Geometry check sheet. Reference: the model listing, model coordinates, mm. A direction names the side the tool comes from. Coordinates: 2 decimals unless noted, no trailing zeros. Loops run counter-clockwise (first coordinate to the right, second up) from the corner with the lowest first, then second, coordinate; pieces in that order, holes last. Notation, with made-up numbers: (-31.5, 16.5) - (3.5, 16.5) arc R9 cw to (3.5, 33.5) - close; hole circle Ø8 at (38, -34). An arc over 180 degrees is marked (long way). Write each question's results on one line, items separated by ' | '. Start each with the question number.
(1) Go/stop test with flat-tipped pins: pin 1 Ø6 at (x, y) = (17.5, 1) entering from -Z; pin 2 Ø5 at (x, y) = (-27.6, 8.005) entering from -Z; pin 3 Ø5 at (x, y) = (-27.6, -8.005) entering from +Z; pin 4 Ø3.5 at (x, y) = (27.6, 8.005) entering from -Z. Record where each tip stops, or that it passes through.
(2) Sectioned sample at B-B (z = 2.75). Enter the section's corners in (x, y).
(3) Sectioned sample at C-C (x = 31.5). Enter the section's corners in (y, z) (3 decimals).
(4) Material ranges on probe 1 along Y at (x, z) = (27.6, 1.35) (3 decimals); probe 2 along X at (y, z) = (-3, 15.25); probe 3 along X at (y, z) = (-6.75, 1), recorded low to high.
(5) Sectioned sample at A-A (x = -18.5). Enter the section's corners in (y, z) (3 decimals).
(6) Mould release check, pull along Z, two halves, no side actions. Record for faces 1 (the face through (-15.58, -6.74, 8.65)), 2 (the face through (-16, 1, 14.5)), 3 (the face through (38.5, 0, 1)), 4 (the face through (15.416, -5.343, 8.091)): pulls with the +Z half, pulls with the -Z half, needs draft (parallel to the pull), parting line crosses it, or undercut.
(7) Access from +Z, -Z, +X, -X, +Y, -Y to the whole of each face (thin tool, end or side, straight path). Record for faces 5 (the face through (15, 1, 14.5)), 6 (the face through (21.5, -3.9, 11.5)), 7 (the face through (15, 1, 16)), 8 (the face through (15.42, 6.09, 7.91)), 9 (the face through (0, 4.13, 1)).
from build123d import *

# Parameters (mm, degrees)
SKETCH1_W                      = 77
SKETCH1_H                      = 20.65
SKETCH1_W_2                    = 66.85
SKETCH1_H_2                    = 8.26
BOSS_EXTRUDE1_DEPTH            = 1.5
CUT_EXTRUDE1_REACH             = 41.889
SKETCH2_R                      = 1.52
CUT_EXTRUDE1_DIRECTION_2_DEPTH = 40.88866537
FILLET1_R                      = 0.76
FILLET1_OF_MIRROR1_R           = 0.76
BOSS_EXTRUDE2_REACH            = 79.704
CUT_EXTRUDE2_START             = -20.65
CUT_EXTRUDE2_OUTLINE_W         = 19
CUT_EXTRUDE2_OUTLINE_H         = 14.5
CUT_EXTRUDE2_OUTLINE_W_2       = 17
CUT_EXTRUDE2_DEPTH             = 20.65
CUT_EXTRUDE3_REACH             = 44.952
SKETCH5_R                      = 0.96


# Read off the part's stored shape, not the designer's step: Mirror2, Cut-Extrude2
with BuildPart() as part:
    # Sketch1 → Boss-Extrude1 (new body)
    with BuildSketch(Plane.XY):
        Rectangle(SKETCH1_W, SKETCH1_H)
        Rectangle(SKETCH1_W_2, SKETCH1_H_2, mode=Mode.SUBTRACT)
    extrude(amount=BOSS_EXTRUDE1_DEPTH)

    # Sketch2 → Cut-Extrude1 (cut, up to next)
    with BuildSketch(Plane.XY.offset(1.5), mode=Mode.PRIVATE) as cut_extrude1_sk1:
        with Locations(Location((-27.6, 8.005, 0), (0, 0, 180))):
            Circle(SKETCH2_R)
    cut_extrude1_tool1 = extrude(cut_extrude1_sk1.sketch, amount=-CUT_EXTRUDE1_REACH, mode=Mode.PRIVATE) & part.part
    cut_extrude1 = cut_extrude1_tool1.solids().sort_by_distance((-27.6, 8.005, 1.5))[0]
    add(cut_extrude1, mode=Mode.SUBTRACT)

    # Sketch2 → Cut-Extrude1 direction 2 (cut)
    with BuildSketch(Plane.XY.offset(1.5)):
        with Locations(Location((-27.6, 8.005, 0), (0, 0, 180))):
            Circle(SKETCH2_R)
    cut_extrude1_direction_2 = extrude(amount=CUT_EXTRUDE1_DIRECTION_2_DEPTH, mode=Mode.SUBTRACT)

    # Fillet1
    fillet1_edges = [part.edges().sort_by_distance(p)[0] for p in [
        (-26.08, 8.005, 0),
    ]]
    fillet(fillet1_edges, radius=FILLET1_R)

    # Mirror1: Cut-Extrude1, Cut-Extrude1 direction 2 across plane
    add(cut_extrude1.mirror(Plane.ZX), mode=Mode.SUBTRACT)
    add(cut_extrude1_direction_2.mirror(Plane.ZX), mode=Mode.SUBTRACT)

    # Fillet1 of Mirror1
    fillet1_of_mirror1_edges = [part.edges().sort_by_distance(p)[0] for p in [
        (-26.08, -8.005, 0),
    ]]
    fillet(fillet1_of_mirror1_edges, radius=FILLET1_OF_MIRROR1_R)

    # Mirror2 outline → Mirror2 (revolve, cut)
    with BuildSketch(Plane(origin=(27.6, 8.005, 0), x_dir=(1, 0, 0), z_dir=(0, -1, 0))):
        with BuildLine():
            Line((1.52, 0.76), (1.52, 1.5))
            Line((1.52, 1.5), (0, 1.5))
            Line((0, 1.5), (0, 0))
            Line((0, 0), (2.28, 0))
            ThreePointArc((2.28, 0), (1.742598846, 0.222598846), (1.52, 0.76))
        make_face()
    revolve(axis=Axis((27.6, 8.005, 0), (0, 0, 1)), mode=Mode.SUBTRACT)

    # Mirror2 2 outline → Mirror2 2 (revolve, cut)
    with BuildSketch(Plane(origin=(27.6, -8.005, 0), x_dir=(1, 0, 0), z_dir=(0, -1, 0))):
        with BuildLine():
            Line((1.52, 0.76), (1.52, 1.5))
            Line((1.52, 1.5), (0, 1.5))
            Line((0, 1.5), (0, 0))
            Line((0, 0), (2.28, 0))
            ThreePointArc((2.28, 0), (1.742598846, 0.222598846), (1.52, 0.76))
        make_face()
    revolve(axis=Axis((27.6, -8.005, 0), (0, 0, 1)), mode=Mode.SUBTRACT)

    # Boss-Extrude2: up to this face of the body (flat: up to its plane)
    boss_extrude2_end = Plane(part.part.faces().sort_by_distance((38.5, 0, 0.75))[0])
    # Sketch3 → Boss-Extrude2 (add, up to the picked face)
    with BuildSketch(Plane.ZY.offset(38.5), mode=Mode.PRIVATE) as boss_extrude2_sk1:
        Polygon((16, 4.410137364), (1.5, 10.325), (1.5, 8.705), (14.5, 3.402019706), (14.5, -2.130032078), (1.5, -8.647068966), (1.5, -10.325), (16, -3.055997317), align=None)
    boss_extrude2_tool1 = split(extrude(boss_extrude2_sk1.sketch, amount=-BOSS_EXTRUDE2_REACH, mode=Mode.PRIVATE), bisect_by=boss_extrude2_end, keep=Keep.BOTH, mode=Mode.PRIVATE)
    add(boss_extrude2_tool1.solids().sort_by(Axis((-38.5, 0.67707, 15.747676), (1, 0, 0)))[0])

    # Cut-Extrude2 outline → Cut-Extrude2 (cut)
    with BuildSketch(Plane(origin=(0, 10.325, 0), x_dir=(1, 0, 0), z_dir=(0, 1, 0)).offset(CUT_EXTRUDE2_START)):
        with Locations((0, -8.75)):
            Rectangle(CUT_EXTRUDE2_OUTLINE_W, CUT_EXTRUDE2_OUTLINE_H)
        with Locations((30, -8.75)):
            Rectangle(CUT_EXTRUDE2_OUTLINE_W_2, CUT_EXTRUDE2_OUTLINE_H)
        with Locations((-30, -8.75)):
            Rectangle(CUT_EXTRUDE2_OUTLINE_W_2, CUT_EXTRUDE2_OUTLINE_H)
    extrude(amount=CUT_EXTRUDE2_DEPTH, mode=Mode.SUBTRACT)

    # Sketch5 → Cut-Extrude3 (cut, up to next)
    with BuildSketch(Plane.XY.offset(16), mode=Mode.PRIVATE) as cut_extrude3_sk1:
        with Locations((-12.5, 0.677070023)):
            Circle(SKETCH5_R)
    cut_extrude3_tool1 = extrude(cut_extrude3_sk1.sketch, amount=-CUT_EXTRUDE3_REACH, mode=Mode.PRIVATE) & part.part
    # Sketch5 → Cut-Extrude3 (cut, up to next)
    with BuildSketch(Plane.XY.offset(16), mode=Mode.PRIVATE) as cut_extrude3_sk2:
        with Locations((-18.5, 0.677070023)):
            Circle(SKETCH5_R)
    cut_extrude3_tool2 = extrude(cut_extrude3_sk2.sketch, amount=-CUT_EXTRUDE3_REACH, mode=Mode.PRIVATE) & part.part
    cut_extrude3_1 = cut_extrude3_tool1.solids().sort_by_distance((-12.5, 0.67707, 16))[0]
    add(cut_extrude3_1, mode=Mode.SUBTRACT)
    cut_extrude3_2 = cut_extrude3_tool2.solids().sort_by_distance((-18.5, 0.67707, 16))[0]
    add(cut_extrude3_2, mode=Mode.SUBTRACT)
    cut_extrude3 = cut_extrude3_1 + cut_extrude3_2  # Cut-Extrude3 as one shape, for the pattern or mirror that repeats it

    # Mirror3: Cut-Extrude3 across plane
    add(cut_extrude3.mirror(Plane(origin=(0, 0, 0), x_dir=(0, 0, 1), z_dir=(1, 0, 0))), mode=Mode.SUBTRACT)


solid = part.part
Outcome:
1) pin 1: stops at z = 13.03 | pin 2: stops at z = 0 | pin 3: stops at z = 1.5 | pin 4: stops at z = 0.22
2) outline: (-21.5, -9.7) - (-9.5, -9.7) - (-9.5, -8.02) - (-21.5, -8.02) - close; (-21.5, 8.2) - (-9.5, 8.2) - (-9.5, 9.82) - (-21.5, 9.82) - close; (9.5, -9.7) - (21.5, -9.7) - (21.5, -8.02) - (9.5, -8.02) - close; (9.5, 8.2) - (21.5, 8.2) - (21.5, 9.82) - (9.5, 9.82) - close
3) outline: (-10.325, 0) - (-4.13, 0) - (-4.13, 1.5) - (-10.325, 1.5) - close; (4.13, 0) - (10.325, 0) - (10.325, 1.5) - (4.13, 1.5) - close
4) probe 1: y = -10.325 to -9.525, -6.485 to -4.13, 4.13 to 6.485, 9.525 to 10.325 | probe 2: x = -21.5 to -9.5, 9.5 to 21.5 | probe 3: x = -38.5 to -28.46, -26.74 to 26.74, 28.46 to 38.5
5) outline: (-10.325, 0) - (-4.13, 0) - (-4.13, 1.5) - (-8.647, 1.5) - (-2.13, 14.5) - (-0.283, 14.5) - (-0.283, 16) - (-3.056, 16) - (-10.325, 1.5) - close; (1.637, 14.5) - (3.402, 14.5) - (8.705, 1.5) - (4.13, 1.5) - (4.13, 0) - (10.325, 0) - (10.325, 1.5) - (4.41, 16) - (1.637, 16) - close
6) face 1: pulls with the +Z half | face 2: pulls with the -Z half | face 3: needs draft | face 4: undercut
7) face 5: -Z, +X, -X | face 6: +Z, +X, +Y, -Y | face 7: +Z, +X, -X, +Y, -Y | face 8: +X, -X | face 9: -Z
